from build123d import *

# Parameters (mm, degrees)
F0_W        = 245
F0_H        = 201
F1_DEPTH    = 8
F2_T        = -2
F3_W        = 210
F3_H        = 174
F4_DEPTH    = 1
F5_W        = 3.5
F5_H        = 33
F6_DEPTH    = 1
F8_W        = 3.5
F8_H        = 4.5
F9_DEPTH    = 1
F10_R       = 2.25
F11_DEPTH   = 1.5
F12_SIZE2   = 1.4896513151
F12_SIZE    = 0.15
F12_2_SIZE2 = 1.4896513151
F12_2_SIZE  = 0.15
F12_3_SIZE2 = 1.4896513151
F12_3_SIZE  = 0.15
F12_4_SIZE2 = 1.4896513151
F12_4_SIZE  = 0.15
F12_5_SIZE2 = 1.4896513151
F12_5_SIZE  = 0.15
F13_R       = 3
F14_DEPTH   = 2.001
F15_W       = 2.5
F15_H       = 1.5
F16_DEPTH   = 245.001
F17_SIZE    = 2
F18_DEPTH   = 2
F19_W       = 186.7508292198
F19_H       = 249.5966032147
F20_DEPTH   = 10.001


with BuildPart() as f1:
    # F0 (on Top) → F1 (new body)
    with BuildSketch(Plane.XY):
        with Locations((122.5, -100.5)):
            Rectangle(F0_W, F0_H)
    extrude(amount=F1_DEPTH)

    # F2
    f2_openings = [f1.faces().sort_by_distance(p)[0] for p in [
        (122.5, -100.5, 8),
    ]]
    offset(amount=F2_T, openings=f2_openings)

    # F3 (on face) → F4 (cut)
    with BuildSketch(Plane.XY.offset(2)):
        with Locations((122.5, -100.5)):
            Rectangle(F3_W, F3_H)
    extrude(amount=-F4_DEPTH, mode=Mode.SUBTRACT)

    # F5 (on face) → F6 (cut)
    with BuildSketch(Plane.XY.offset(2)):
        with Locations((6.25, -27.5)):
            Rectangle(F5_W, F5_H)
        with Locations((6.25, -173.5)):
            Rectangle(F5_W, F5_H)
        with Locations((238.75, -27.5)):
            Rectangle(F5_W, F5_H)
        with Locations((238.75, -173.5)):
            Rectangle(F5_W, F5_H)
    extrude(amount=-F6_DEPTH, mode=Mode.SUBTRACT)

    # F8 (on face) → F9 (join)
    with BuildSketch(Plane.XY.offset(2)):
        with Locations((238.75, -173.5)):
            Rectangle(F8_W, F8_H)
        with Locations((238.75, -27.5)):
            Rectangle(F8_W, F8_H)
        with Locations((6.25, -27.5)):
            Rectangle(F8_W, F8_H)
        with Locations((6.25, -173.5)):
            Rectangle(F8_W, F8_H)
    extrude(amount=-F9_DEPTH)

    # F10 (on face) → F11 (join)
    with BuildSketch(Plane.XY.offset(2)):
        with Locations((238.5, -27.5)):
            Circle(F10_R)
        with Locations((6.5, -27.5)):
            Circle(F10_R)
        with Locations((6.5, -173.5)):
            Circle(F10_R)
        with Locations((238.5, -173.5)):
            Circle(F10_R)
        with Locations((122.5, -8.5)):
            Circle(F10_R)
    extrude(amount=F11_DEPTH)

    # F12
    f12_edges = [f1.edges().sort_by_distance(p)[0] for p in [
        (236.25, -173.5, 3.5),
    ]]
    f12_side = f1.faces().sort_by_distance((238.5, -173.5, 3.5))[0]
    chamfer(f12_edges, length=F12_SIZE, length2=F12_SIZE2, reference=f12_side)

    # F12#2
    f12_2_edges = [f1.edges().sort_by_distance(p)[0] for p in [
        (4.25, -173.5, 3.5),
    ]]
    f12_2_side = f1.faces().sort_by_distance((6.5, -173.5, 3.5))[0]
    chamfer(f12_2_edges, length=F12_2_SIZE, length2=F12_2_SIZE2, reference=f12_2_side)

    # F12#3
    f12_3_edges = [f1.edges().sort_by_distance(p)[0] for p in [
        (236.25, -27.5, 3.5),
    ]]
    f12_3_side = f1.faces().sort_by_distance((238.5, -27.5, 3.5))[0]
    chamfer(f12_3_edges, length=F12_3_SIZE, length2=F12_3_SIZE2, reference=f12_3_side)

    # F12#4
    f12_4_edges = [f1.edges().sort_by_distance(p)[0] for p in [
        (4.25, -27.5, 3.5),
    ]]
    f12_4_side = f1.faces().sort_by_distance((6.5, -27.5, 3.5))[0]
    chamfer(f12_4_edges, length=F12_4_SIZE, length2=F12_4_SIZE2, reference=f12_4_side)

    # F12#5
    f12_5_edges = [f1.edges().sort_by_distance(p)[0] for p in [
        (120.25, -8.5, 3.5),
    ]]
    f12_5_side = f1.faces().sort_by_distance((122.5, -8.5, 3.5))[0]
    chamfer(f12_5_edges, length=F12_5_SIZE, length2=F12_5_SIZE2, reference=f12_5_side)

    # F13 (on face) → F14 (cut, through all)
    with BuildSketch(Plane.XY.offset(2)):
        with Locations((7, -54.5)):
            Circle(F13_R)
        with Locations((7, -100.5)):
            Circle(F13_R)
        with Locations((7, -146.5)):
            Circle(F13_R)
        with Locations((238, -54.5)):
            Circle(F13_R)
        with Locations((238, -100.5)):
            Circle(F13_R)
        with Locations((238, -146.5)):
            Circle(F13_R)
        with Locations((87.3, -8.5)):
            Circle(F13_R)
        with Locations((87.3, -67.5)):
            Circle(F13_R)
        with Locations((157.7, -8.5)):
            Circle(F13_R)
        with Locations((157.7, -67.5)):
            Circle(F13_R)
        with Locations((157.7, -133.5)):
            Circle(F13_R)
        with Locations((157.7, -192.5)):
            Circle(F13_R)
        with Locations((87.3, -192.5)):
            Circle(F13_R)
        with Locations((87.3, -133.5)):
            Circle(F13_R)
    extrude(amount=-F14_DEPTH, mode=Mode.SUBTRACT)

    # F15 (on face) → F16 (cut, through all)
    with BuildSketch(Plane(origin=(0, 0, 0), x_dir=(0, -1, 0), z_dir=(-1, 0, 0))):
        with Locations((1.25, 0.75)):
            Rectangle(F15_W, F15_H)
        with Locations((199.75, 0.75)):
            Rectangle(F15_W, F15_H)
    extrude(amount=-F16_DEPTH, mode=Mode.SUBTRACT)

    # F17
    f17_edges = [f1.edges().sort_by_distance(p)[0] for p in [
        (122.5, -2, 2),
        (122.5, -199, 2),
    ]]
    chamfer(f17_edges, length=F17_SIZE)

    # F18 (add): a face of the model
    f18_faces = [f1.faces().sort_by_distance(p)[0] for p in [
        (122.5, -0.3169006153, 8),
    ]]
    extrude(f18_faces, amount=F18_DEPTH)

    # F19 (on face) → F20 (cut, through all)
    with BuildSketch(Plane(origin=(0, 0, 0), x_dir=(1, 0, 0), z_dir=(0, 0, -1))):
        with Locations((211.746044457, 104.012247175)):
            Rectangle(F19_W, F19_H)
    extrude(amount=-F20_DEPTH, mode=Mode.SUBTRACT)


solid = f1.part
CAD build for the part. Positions are in the model's coordinates, mm. A direction names the side the tool comes from. Round coordinates to 2 decimals unless told otherwise and drop trailing zeros. Loops run counter-clockwise (first coordinate to the right, second up) from the corner with the lowest first, then second, coordinate; pieces in that order, holes last.
(1) Cut at C-C (y = -181). Give the cut face in (x, z).
(2) Which spindle directions (+Z, -Z, +X, -X, +Y, -Y) get a long thin tool onto all of the face, cutting with end or side? Do faces 1 (the cylindrical face through (88.91, -130.97, 0.51)), 2 (the flat face through (6, -173, 3.5)). Say none if no direction does.
(3) Wall check: line 1 along Y through (x, z) = (87.3, 0.2); line 2 along Y through (x, z) = (87.3, 1.3); line 3 along Y through (x, z) = (70, 5.25). Give the ranges that are in metal, low to high.
(4) Drop flat-ended pins along their axis: pin 1 (4.5 mm diameter, centred on x = 7, y = -174, fed in from +Z); pin 2 (5 mm diameter, centred on x = 7, y = -100.5, fed in from -Z); pin 3 (3 mm diameter, centred on x = 7, y = -20.5, fed in from +Z); pin 4 (0.8 mm diameter, centred on y = -17.5, z = 1.5, fed in from +X). Give the stop position or say it passes through.
(5) Two-plate mould, pull along Y, no slides. Class faces 3 (the flat face through (118.371, -100, 0.5)), 4 (the flat face through (58, 0, 6)), 5 (the flat face through (59, -199, 7)), 6 (the flat face through (58, -201, 6)): +Y half, -Y half, draft (parallel to the pull), parting line (faces both ways), or undercut.
(6) Cut at B-B (y = -67.5). Give the cut face in (x, z), plus the area to 3 significant figures.
(7) Cut at A-A (x = 87.3). State how many separate pieces and enclosed holes the cut face has, plus the area to 4 significant figures.
(8) Cut at D-D (z = 8). Give the cut face in (x, y).
Findings below:
1. outline: (0, 0) - (118.37, 0) - (118.37, 1) - (17.5, 1) - (17.5, 2) - (8, 2) - (8, 1) - (4.5, 1) - (4.5, 2) - (2, 2) - (2, 10) - (0, 10) - close
2. face 1: +Z, -Z
2. face 2: +Z, +X
3. line 1: y = -198.5 to -195.5, -189.5 to -136.5, -130.5 to -70.5, -64.5 to -11.5, -5.5 to -2.5
3. line 2: y = -198.5 to -195.5, -189.5 to -187.5, -13.5 to -11.5, -5.5 to -2.5
3. line 3: y = -201 to -199, -2 to 0
4. pin 1: stops at z = 3.5
4. pin 2: passes through
4. pin 3: stops at z = 2
4. pin 4: stops at x = 17.5
5. face 3: draft
5. face 4: +Y half
5. face 5: undercut
5. face 6: -Y half
6. outline: (0, 0) - (84.3, 0) - (84.3, 1) - (17.5, 1) - (17.5, 2) - (2, 2) - (2, 10) - (0, 10) - close; (90.3, 0) - (118.37, 0) - (118.37, 1) - (90.3, 1) - close
6. area: 146 mm2
7. separate pieces: 5
7. enclosed holes: 0
7. area: 220.5 mm2
8. outline: (0, -201) - (118.37, -201) - (118.37, -199) - (2, -199) - (2, -2) - (118.37, -2) - (118.37, 0) - (0, 0) - close
